Check sheet for the modelled part. Datum: model origin and axes. Units: mm. Round coordinates to 2 decimals unless told otherwise and drop trailing zeros.
Item 1: Cross-section at A-A on z = 674. Count the separate pieces of the cut face and the enclosed holes in it, plus the area to 3 significant figures.
Item 2: Material ranges on line 1 (Y direction, x = 0, z = 332.5); line 2 (X direction, y = -4, z = 240.5); line 3 (X direction, y = -5, z = 724.5), recorded low to high.
Item 3: Go/stop test with flat-tipped pins: pin 1 Ø8 at (y, z) = (12, 537) entering from +X; pin 2 Ø0.6 at (x, z) = (-13.5, 799) entering from -Y; pin 3 Ø8 at (x, z) = (-1, 219) entering from +Y; pin 4 Ø3 at (x, z) = (-1, 330.5) entering from -Y. Record where each tip stops, or that it passes through.
from build123d import *

# Parameters (mm, degrees)
CROQUIS1_R              = 3.35
SALIENTE_EXTRUIR1_DEPTH = 1200
REDONDEO1_R             = 1.5


with BuildPart() as part:
    # Croquis1 → Saliente-Extruir1 (new body)
    with BuildSketch(Plane.XY):
        with BuildLine():
            Line((-12.05, -30.05), (-4, -30.05))
            Line((-4, -30.05), (-4, -27.75))
            Line((-4, -27.75), (-11.7, -27.75))
            Line((-11.7, -27.75), (-5, -21.05))
            Line((-5, -21.05), (5, -21.05))
            Line((5, -21.05), (11.7, -27.75))
            Line((11.7, -27.75), (4, -27.75))
            Line((4, -27.75), (4, -30.05))
            Line((4, -30.05), (12.05, -30.05))
            ThreePointArc((12.05, -30.05), (14.171320344, -29.171320344), (15.05, -27.05))
            Line((15.05, -27.05), (15.05, -18.55))
            Line((15.05, -18.55), (12.75, -18.55))
            Line((12.75, -18.55), (12.75, -25.8))
            Line((12.75, -25.8), (6.5, -19.55))
            Line((6.5, -19.55), (6.5, -9.55))
            Line((6.5, -9.55), (12.75, -3.3))
            Line((12.75, -3.3), (12.75, -10.55))
            Line((12.75, -10.55), (15.05, -10.55))
            Line((15.05, -10.55), (15.05, 10.55))
            Line((15.05, 10.55), (12.75, 10.55))
            Line((12.75, 10.55), (12.75, 3.3))
            Line((12.75, 3.3), (6.5, 9.55))
            Line((6.5, 9.55), (6.5, 19.55))
            Line((6.5, 19.55), (12.75, 25.8))
            Line((12.75, 25.8), (12.75, 18.55))
            Line((12.75, 18.55), (15.05, 18.55))
            Line((15.05, 18.55), (15.05, 27.05))
            ThreePointArc((15.05, 27.05), (14.171320344, 29.171320344), (12.05, 30.05))
            Line((12.05, 30.05), (4, 30.05))
            Line((4, 30.05), (4, 27.75))
            Line((4, 27.75), (11.7, 27.75))
            Line((11.7, 27.75), (5, 21.05))
            Line((5, 21.05), (-5, 21.05))
            Line((-5, 21.05), (-11.7, 27.75))
            Line((-11.7, 27.75), (-4, 27.75))
            Line((-4, 27.75), (-4, 30.05))
            Line((-4, 30.05), (-12.05, 30.05))
            ThreePointArc((-12.05, 30.05), (-14.171320344, 29.171320344), (-15.05, 27.05))
            Line((-15.05, 27.05), (-15.05, 18.55))
            Line((-15.05, 18.55), (-12.75, 18.55))
            Line((-12.75, 18.55), (-12.75, 25.8))
            Line((-12.75, 25.8), (-6.5, 19.55))
            Line((-6.5, 19.55), (-6.5, 9.55))
            Line((-6.5, 9.55), (-12.75, 3.3))
            Line((-12.75, 3.3), (-12.75, 10.55))
            Line((-12.75, 10.55), (-15.05, 10.55))
            Line((-15.05, 10.55), (-15.05, -10.55))
            Line((-15.05, -10.55), (-12.75, -10.55))
            Line((-12.75, -10.55), (-12.75, -3.3))
            Line((-12.75, -3.3), (-6.5, -9.55))
            Line((-6.5, -9.55), (-6.5, -19.55))
            Line((-6.5, -19.55), (-12.75, -25.8))
            Line((-12.75, -25.8), (-12.75, -18.55))
            Line((-12.75, -18.55), (-15.05, -18.55))
            Line((-15.05, -18.55), (-15.05, -27.05))
            ThreePointArc((-15.05, -27.05), (-14.171320344, -29.171320344), (-12.05, -30.05))
        make_face()
        with Locations((0, 14.55)):
            Circle(CROQUIS1_R, mode=Mode.SUBTRACT)
        with Locations((0, -14.55)):
            Circle(CROQUIS1_R, mode=Mode.SUBTRACT)
        Polygon((-5, 8.05), (5, 8.05), (11.7, 1.35), (12.75, 0.3), (12.75, -0.3), (11.7, -1.35), (5, -8.05), (-5, -8.05), (-11.7, -1.35), (-12.75, -0.3), (-12.75, 0.3), (-11.7, 1.35), align=None, mode=Mode.SUBTRACT)
    extrude(amount=SALIENTE_EXTRUIR1_DEPTH)

    # Redondeo1
    redondeo1_edges = [part.edges().sort_by_distance(p)[0] for p in [
        (-4, 30.05, 600),
        (4, 30.05, 600),
        (15.05, 18.55, 600),
        (15.05, 10.55, 600),
        (15.05, -10.55, 600),
        (15.05, -18.55, 600),
        (4, -30.05, 600),
        (-4, -30.05, 600),
        (-15.05, -18.55, 600),
        (-15.05, -10.55, 600),
        (-15.05, 10.55, 600),
        (-15.05, 18.55, 600),
    ]]
    fillet(redondeo1_edges, radius=REDONDEO1_R)


solid = part.part
Response values:
1. separate pieces: 1
1. enclosed holes: 3
1. area: 694 mm2
2. line 1: y = -21.05 to -17.9, -11.2 to -8.05, 8.05 to 11.2, 17.9 to 21.05
2. line 2: x = -15.05 to -12.75, -12.05 to -9.05, 9.05 to 12.05, 12.75 to 15.05
2. line 3: x = -15.05 to -12.75, -11.05 to -8.05, 8.05 to 11.05, 12.75 to 15.05
3. pin 1: stops at x = 15.05
3. pin 2: stops at y = -29.82
3. pin 3: stops at y = 29.96
3. pin 4: stops at y = -21.05
